Design review of the part built by this model. Coordinates are the model's own, in mm. A direction names the side the tool comes from. Coordinates: 2 decimals unless noted, no trailing zeros. Loops run counter-clockwise (first coordinate to the right, second up) from the corner with the lowest first, then second, coordinate; pieces in that order, holes last. Notation, with made-up numbers: M 37.5,13.5 L 66.5,13.5 A29 ccw 66.5,43.5 Z; hole C -11.75,0.5 d4. An arc over 180 degrees is marked long. Put each result on its own line as item: value. Start each with the question number.
(1) Take a section at B-B, the plane y = 11. Give the boundary of the cut face in (x, z), then the cut area to 3 significant figures.
(2) Take a section at C-C, the plane z = 2.3. Give the boundary of the cut face in (x, y).
(3) For probe 1 along Y at (x, z) = (10, 2.85); probe 2 along X at (y, z) = (-18.5, 2.1); probe 3 along Y at (x, z) = (-33.5, 1.85), list the stretches that pass through material, from the lowest coordinate up. Write a range as [from, to].
(4) Take a section at A-A, the plane x = -26. Give the boundary of the cut face in (y, z).
(5) For faces 1 (the flat face through (-2, -57, 1)), 2 (the flat face through (-2, 57, 1)), 3 (the flat face through (7, -40, 3)), 4 (the flat face through (5, -51, 1)), 5 (the flat face through (3, 55, 1)), list the 3-axis set-ups (+Z, -Z, +X, -X, +Y, -Y) from which the entire face can be reached by the end or side of a thin tool; tool diameter is ignored.
(6) Clearance check with flat-ended pins moving along their axes: pin 1 (0.9 mm diameter, centred on y = 50, z = 1, fed in from -X); pin 2 (0.9 mm diameter, centred on y = 52, z = 1, fed in from +X); pin 3 (1.5 mm diameter, centred on y = 57, z = 1.5, fed in from +X). State where each tip first meets the part, or that it passes through.
(7) Take a section at D-D, the plane y = -45.5. Give the boundary of the cut face in (x, z), then the cut area to 3 significant figures.
```python
from build123d import *

# Parameters (mm, degrees)
PAD_DEPTH            = 3
PAD_MIRRORED_2_DEPTH = 3


with BuildPart() as part:
    # Sketch → Pad (new body)
    with BuildSketch(Plane.XY):
        with BuildLine():
            ThreePointArc((47.5, 0), (35.311117, 31.770663), (5, 47.236109))
            Line((5, 55), (5, 47.236109))
            Line((2, 55), (5, 55))
            Line((2, 55), (2, 59))
            Line((2, 59), (0, 59))
            Line((0, 40), (0, 59))
            ThreePointArc((40, 0), (28.284271, 28.284271), (0, 40))
            Line((40, 0), (47.5, 0))
        make_face()
    pad = extrude(amount=PAD_DEPTH)

    # Sketch Mirrored 2 → Pad Mirrored 2 (add)
    with BuildSketch(Plane(origin=(0, 0, 0), x_dir=(-1, 0, 0), z_dir=(0, 0, -1))):
        with BuildLine():
            ThreePointArc((47.5, 0), (35.311117, 31.770663), (5, 47.236109))
            Line((5, 55), (5, 47.236109))
            Line((2, 55), (5, 55))
            Line((2, 55), (2, 59))
            Line((2, 59), (0, 59))
            Line((0, 40), (0, 59))
            ThreePointArc((40, 0), (28.284271, 28.284271), (0, 40))
            Line((40, 0), (47.5, 0))
        make_face()
    pad_mirrored_2 = extrude(amount=-PAD_MIRRORED_2_DEPTH)

    # Mirrored001: Pad, Pad Mirrored 2 across Sketch H_Axis
    add(pad.mirror(Plane.ZX))
    add(pad_mirrored_2.mirror(Plane.ZX))


solid = part.part
```
Computed values:
1. outline: M -46.21,0 L -38.46,0 L -38.46,3 L -46.21,3 Z; M 38.46,0 L 46.21,0 L 46.21,3 L 38.46,3 Z
1. area: 46.5 mm^2
2. outline: M -5,-55 L -2,-55 L -2,-59 L 2,-59 L 2,-55 L 5,-55 L 5,-47.24 A47.5 ccw 5,47.24 L 5,55 L 2,55 L 2,59 L -2,59 L -2,55 L -5,55 L -5,47.24 A47.5 ccw -5,-47.24 Z; hole M -40,0 A40 ccw 0,-40 A40 ccw 40,0 A40 ccw 0,40 A40 ccw Z
3. probe 1: y = [-46.44, -38.73], [38.73, 46.44]
3. probe 2: x = [-43.75, -35.46], [35.46, 43.75]
3. probe 3: y = [-33.67, -21.86], [21.86, 33.67]
4. outline: M -39.75,0 L -30.4,0 L -30.4,3 L -39.75,3 Z; M 30.4,0 L 39.75,0 L 39.75,3 L 30.4,3 Z
5. face 1: +Z, -Z, -X, -Y
5. face 2: +Z, -Z, -X, +Y
5. face 3: +Z, +X, -X, +Y, -Y
5. face 4: +Z, -Z, +X, -Y
5. face 5: +Z, -Z, +X, +Y
6. pin 1: stops at x = -5
6. pin 2: stops at x = 5
6. pin 3: stops at x = 2
7. outline: M -13.64,0 L 13.64,0 L 13.64,3 L -13.64,3 Z
7. area: 81.8 mm^2
